Could you check a few things on this model? Use its own coordinates, in mm. A direction names the side the tool comes from. Round coordinates to 2 decimals unless told otherwise and drop trailing zeros. Write each loop counter-clockwise with the first axis right and the second up, starting at its lowest first coordinate (ties: lowest second). Pieces come first, ordered by that corner, then holes. Notation, with made-up numbers: (-6, 84.25) -> (40, 84.25) arc R25 cw to (40, 118.25) -> close; hole circle Ø1 at (66.5, 77). An arc over 180 degrees is marked (long way). Return JSON: item names as keys, results as strings.
from build123d import *

# Parameters (mm, degrees)
BLANKSKE_W        = 62.5
BLANKSKE_H        = 13.25
BLANKSKE_R        = 2
BLANK_DEPTH       = 5
TOOTHCUTSIM_DEPTH = 65.084416983
TEETHCUTS_COUNT   = 17
TEETHCUTS_PITCH   = 3.926990813
FILLET1_R         = 3


with BuildPart() as part:
    # BlankSke → Blank (new body)
    with BuildSketch(Plane.XY):
        with Locations((31.25, 6.625)):
            Rectangle(BLANKSKE_W, BLANKSKE_H)
        with Locations((4, 5.5)):
            Circle(BLANKSKE_R, mode=Mode.SUBTRACT)
        with Locations(Location((58.5, 5.5, 0), (0, 0, 180))):
            Circle(BLANKSKE_R, mode=Mode.SUBTRACT)
    extrude(amount=-BLANK_DEPTH)

    # TooCutSkeSim → ToothCutSim (cut, through all)
    with BuildSketch(Plane.XY):
        Polygon((0.548044212, 10.4375), (-0.548044212, 10.4375), (-1.58095534, 13.2754), (1.58095534, 13.2754), align=None)
    toothcutsim = extrude(amount=-TOOTHCUTSIM_DEPTH, mode=Mode.SUBTRACT)

    # TeethCuts: ToothCutSim ×17
    with Locations(*[(i * TEETHCUTS_PITCH, 0, 0) for i in range(1, TEETHCUTS_COUNT)]):
        add(toothcutsim, mode=Mode.SUBTRACT)

    # Fillet1
    fillet1_edges = [part.edges().sort_by_distance(p)[0] for p in [
        (62.5, 0, -2.5),
        (0, 0, -2.5),
    ]]
    fillet(fillet1_edges, radius=FILLET1_R)


solid = part.part
1) Thinking about a two-plate mould opening in X: for faces 3 (the face through (61.78, 11.82, -2.46)), 4 (the face through (59, 10.438, -2)), 5 (the face through (31, 7, 0)), which applies, pulls with the +X half, pulls with the -X half, needs draft (parallel to the pull), parting line crosses it, or undercut?
Return value:
{"face 3": "pulls with the +X half", "face 4": "undercut", "face 5": "needs draft"}
2) I want a section at C-C, the plane y = 1.25. Please give me the cut outline in (x, z), and give its area (3 significant figures).
Return value:
{"outline": "(0.56, -5) -> (61.94, -5) -> (61.94, 0) -> (0.56, 0) -> close", "area": "307 mm²"}
3) Will these pins go through, and if not, where does the flat tip stop? pin 1 Ø3 at (y, z) = (12, -4) entering from +X; pin 2 Ø0.9 at (x, z) = (23.5, -2.5) entering from +Y.
Return value:
{"pin 1": "x = 62.26", "pin 2": "y = 10.44"}
4) If I drill on probe 1 along X at (y, z) = (5.75, -0.7); probe 2 along Y at (x, z) = (58.5, -1); probe 3 along X at (y, z) = (6.25, -4.1), over which ranges is the centre line in solid material (lowest first)? Write a range as [from, to].
Return value:
{"probe 1": "[0, 2.02], [5.98, 56.52], [60.48, 62.5]", "probe 2": "[0, 3.5], [7.5, 10.44]", "probe 3": "[0, 2.15], [5.85, 56.65], [60.35, 62.5]"}
5) I want a section at B-B, the plane z = -2.35. Count the separate pieces of the cut face and the enclosed holes in it, and give its area (3 significant figures).
Return value:
{"separate pieces": "1", "enclosed holes": "2", "area": "705 mm²"}
6) For faces 1 (the face through (0, 7, -2)), 2 (the face through (14.655, 11.824, -2.465)), which set-ups out of +Z, -Z, +X, -X, +Y, -Y let a thin tool reach every point of the face, with its end or its side?
Return value:
{"face 1": "+Z, -Z, -X, +Y, -Y", "face 2": "+Z, -Z, +Y"}
7) I want a section at A-A, the plane y = 5.5. Please give me the cut outline in (x, z).
Return value:
{"outline": "(0, -5) -> (2, -5) -> (2, 0) -> (0, 0) -> close; (6, -5) -> (56.5, -5) -> (56.5, 0) -> (6, 0) -> close; (60.5, -5) -> (62.5, -5) -> (62.5, 0) -> (60.5, 0) -> close"}
